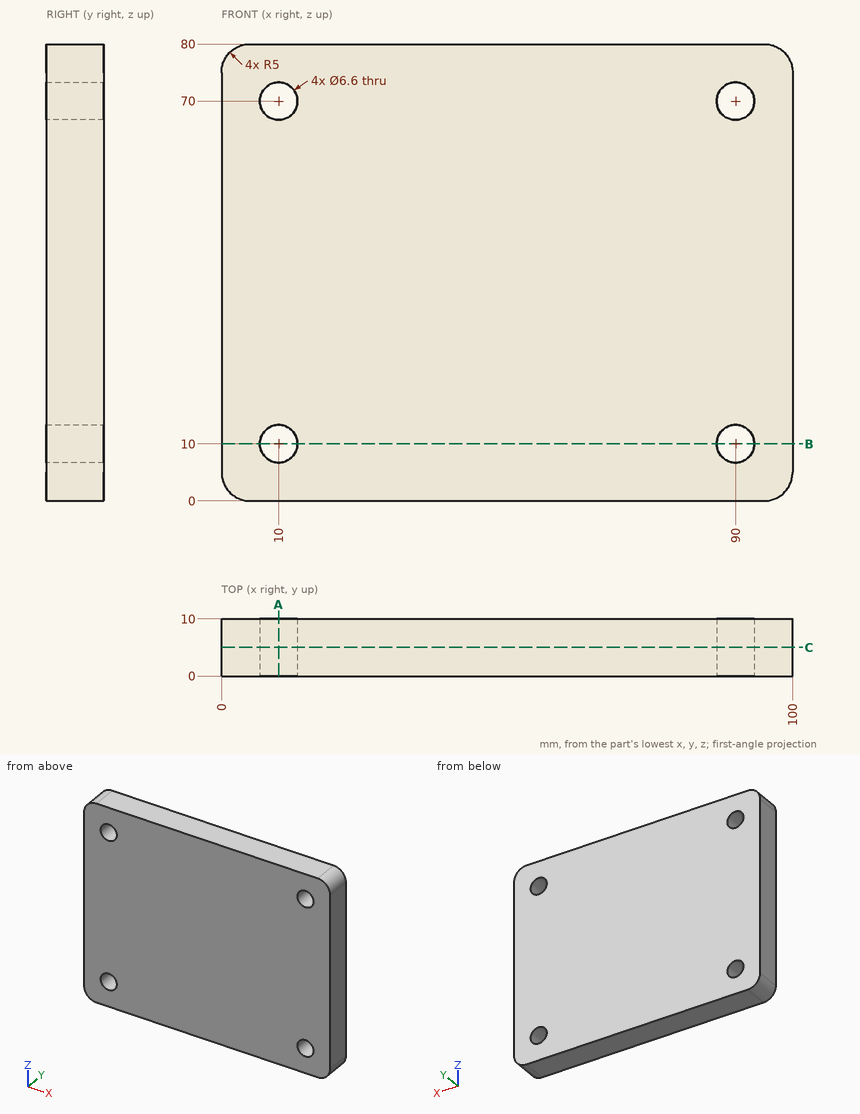
Could you check a few things on this drawing? It's one solid part, dimensions in mm from its lowest x, y, z. Coordinates: 2 decimals unless noted, no trailing zeros. Order: outer loops, then holes, each group sorted by start corner. A loop starts at its lowest first (then second) coordinate and runs counter-clockwise, first axis right, second up. Notation, with made-up numbers: M -32,6 L 0,6 A11 ccw 0,27 Z; hole C 67.25,-9.5 d4. An arc over 180 degrees is marked long. Use a Markdown table: item, result. Add a question column.
Q1. I want a section at A-A on x = 10. List the corners of the cut face in (y, z) for me.
Q2. I want a section at C-C on y = 5. List the corners of the cut face in (x, z) for me.
Q3. If I drill on L1, parallel to X at y = 5.5, z = 70; L2, parallel to Z at x = 10, y = 2.25; L3, parallel to X at y = 0.5, z = 72, over which ranges is the centre line in solid material (lowest first)?
Q4. I want a section at B-B on z = 10. List the corners of the cut face in (x, y) for me.
Checked values:
| question | item | result |
|---|---|---|
| 1 | outline | M 0,0 L 10,0 L 10,6.7 L 0,6.7 Z; M 0,13.3 L 10,13.3 L 10,66.7 L 0,66.7 Z; M 0,73.3 L 10,73.3 L 10,80 L 0,80 Z |
| 2 | outline | M 0,5 A5 ccw 5,0 L 95,0 A5 ccw 100,5 L 100,75 A5 ccw 95,80 L 5,80 A5 ccw 0,75 Z; hole C 10,10 d6.6; hole C 10,70 d6.6; hole C 90,10 d6.6; hole C 90,70 d6.6 |
| 3 | L1 | 0 to 6.7, 13.3 to 86.7, 93.3 to 100 |
| 3 | L2 | 0 to 6.7, 13.3 to 66.7, 73.3 to 80 |
| 3 | L3 | 0 to 7.38, 12.62 to 87.38, 92.62 to 100 |
| 4 | outline | M 0,0 L 6.7,0 L 6.7,10 L 0,10 Z; M 13.3,0 L 86.7,0 L 86.7,10 L 13.3,10 Z; M 93.3,0 L 100,0 L 100,10 L 93.3,10 Z |
